The listing builds one solid part. Answer for the finished solid, in the listing's coordinates (mm). Face numbers are marked on the shaded views. A direction names the side the tool comes from. Give positions to 0.01 mm unless a question says otherwise; leave off trailing zeros. Write each loop counter-clockwise with the first axis right and the second up, starting at its lowest first coordinate (ties: lowest second). Pieces come first, ordered by that corner, then holes. Notation, with made-up numbers: M 72,-0.75 L 107,-0.75 A18 ccw 107,28.25 Z; hole C 64.25,-9 d3. An arc over 180 degrees is marked long. Return JSON: item names as keys, results as strings.
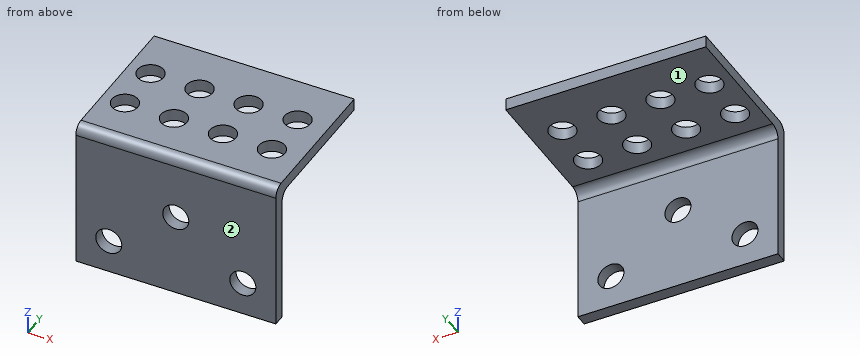
from build123d import *

# Parameters (mm, degrees)
BOSS_EXTRUDE2_DEPTH = 40
SKETCH1_R           = 2.6
CUT_EXTRUDE4_DEPTH  = 40
SKETCH5_R           = 2.6
CUT_EXTRUDE5_DEPTH  = 40


with BuildPart() as part:
    # Sketch3 → Boss-Extrude2 (new body)
    with BuildSketch(Plane(origin=(0, 0, 0), x_dir=(0, 0, -1), z_dir=(1, 0, 0))):
        with BuildLine():
            Line((2, -17.949216757), (29.9, -17.949216757))
            Line((29.9, -17.949216757), (29.9, -15.549216757))
            Line((29.9, -15.549216757), (4.4, -15.549216757))
            ThreePointArc((4.4, -15.549216757), (2.985786438, -14.963430319), (2.4, -13.549216757))
            Line((2.4, -13.549216757), (2.4, 12.010783243))
            Line((2.4, 12.010783243), (0, 12.010783243))
            Line((0, 12.010783243), (0, -15.949216757))
            ThreePointArc((0, -15.949216757), (0.585786438, -17.363430319), (2, -17.949216757))
        make_face()
    extrude(amount=-BOSS_EXTRUDE2_DEPTH)

    # Sketch1 → Cut-Extrude4 (cut)
    with BuildSketch(Plane.XY):
        with Locations((-35.455799348, 1.940783243)):
            Circle(SKETCH1_R)
        with Locations((-25.655799348, 1.940783243)):
            Circle(SKETCH1_R)
        with Locations((-15.855799348, 1.940783243)):
            Circle(SKETCH1_R)
        with Locations((-6.055799348, 1.940783243)):
            Circle(SKETCH1_R)
        with Locations(Location((-6.055799348, -7.859216757, 0), (0, 0, 180))):  # turned: the seam where the file's is
            Circle(SKETCH1_R)
        with Locations(Location((-15.855799348, -7.859216757, 0), (0, 0, 180))):  # turned: the seam where the file's is
            Circle(SKETCH1_R)
        with Locations(Location((-25.655799348, -7.859216757, 0), (0, 0, 180))):  # turned: the seam where the file's is
            Circle(SKETCH1_R)
        with Locations(Location((-35.455799348, -7.859216757, 0), (0, 0, 180))):  # turned: the seam where the file's is
            Circle(SKETCH1_R)
    extrude(amount=-CUT_EXTRUDE4_DEPTH, mode=Mode.SUBTRACT)

    # Sketch5 → Cut-Extrude5 (cut)
    with BuildSketch(Plane(origin=(0, -15.549216757, 0), x_dir=(1, 0, 0), z_dir=(0, 1, 0))):
        with Locations(Location((-33.4, 23.2, 0), (0, 0, 270))):  # turned: the seam where the file's is
            Circle(SKETCH5_R)
        with Locations(Location((-6.6, 23.2, 0), (0, 0, 90))):  # turned: the seam where the file's is
            Circle(SKETCH5_R)
        with Locations(Location((-20, 13.2, 0), (0, 0, 270))):  # turned: the seam where the file's is
            Circle(SKETCH5_R)
    extrude(amount=-CUT_EXTRUDE5_DEPTH, mode=Mode.SUBTRACT)


solid = part.part
Item 1: Find the intervals of material crossed by line 1 (X direction, y = -16.2, z = -23.2); line 2 (X direction, y = -9, z = -2); line 3 (Y direction, x = -38, z = -10.25), in increasing order.
Geometry results:
{"line 1": "x = -40 to -36, -30.8 to -9.2, -4 to 0", "line 2": "x = -40 to -37.79, -33.12 to -27.99, -23.32 to -18.19, -13.52 to -8.39, -3.72 to 0", "line 3": "y = -17.95 to -15.55"}
Item 2: A cutting plane is placed at B-B, the plane z = -13.2. Write down the section's boundary in (x, y).
Geometry results:
{"outline": "M -40,-17.95 L -22.6,-17.95 L -22.6,-15.55 L -40,-15.55 Z; M -17.4,-17.95 L 0,-17.95 L 0,-15.55 L -17.4,-15.55 Z"}
Item 3: Given pin 1 Ø12 at (y, z) = (-1, -12.5) entering from -X; pin 2 Ø12 at (x, y) = (-32, 8.5) entering from -Z; pin 3 Ø7 at (x, z) = (-6.6, -23.2) entering from +Y; pin 4 Ø8 at (x, z) = (-27.5, -7) entering from +Y, each flat-ended and moving along its own axis, determine where each tip first touches the part or whether it passes through.
Geometry results:
{"pin 1": "passes through", "pin 2": "stops at z = -2.4", "pin 3": "stops at y = -15.55", "pin 4": "stops at y = -14.98"}
Item 4: A cutting plane is placed at C-C, the plane x = -20. Write down the section's boundary in (y, z).
Geometry results:
{"outline": "M -17.95,-29.9 L -15.55,-29.9 L -15.55,-15.8 L -17.95,-15.8 Z; M -17.95,-10.6 L -15.55,-10.6 L -15.55,-4.4 A2 cw -13.55,-2.4 L 12.01,-2.4 L 12.01,0 L -15.95,0 A2 ccw -17.95,-2 Z"}
Item 5: A cutting plane is placed at D-D, the plane x = -36.5. Write down the section's boundary in (y, z), plus the area to 3 significant figures.
Geometry results:
{"outline": "M -17.95,-29.9 L -15.55,-29.9 L -15.55,-4.4 A2 cw -13.55,-2.4 L -10.24,-2.4 L -10.24,0 L -15.95,0 A2 ccw -17.95,-2 Z; M -5.48,-2.4 L -0.44,-2.4 L -0.44,0 L -5.48,0 Z; M 4.32,-2.4 L 12.01,-2.4 L 12.01,0 L 4.32,0 Z", "area": "115 mm2"}
Item 6: A cutting plane is placed at A-A, the plane z = -23.2. Write down the section's boundary in (x, y).
Geometry results:
{"outline": "M -40,-17.95 L -36,-17.95 L -36,-15.55 L -40,-15.55 Z; M -30.8,-17.95 L -9.2,-17.95 L -9.2,-15.55 L -30.8,-15.55 Z; M -4,-17.95 L 0,-17.95 L 0,-15.55 L -4,-15.55 Z"}
Item 7: Which of the six approach directions +Z, -Z, +X, -X, +Y, -Y give full straight-line access (tool end or side, diameter ignored) to the marked faces 1 and 2?
Geometry results:
{"face 1": "-Z, +X, -X, +Y", "face 2": "+Z, -Z, +X, -X, -Y"}
